Input: dimensioned drawing with shaded views. Units: mm. Origin: part minimum x, y, z. A direction names the side the tool comes from. Coordinates: 2 decimals unless noted, no trailing zeros. Order: outer loops, then holes, each group sorted by start corner. A loop starts at its lowest first (then second) coordinate and runs counter-clockwise, first axis right, second up.
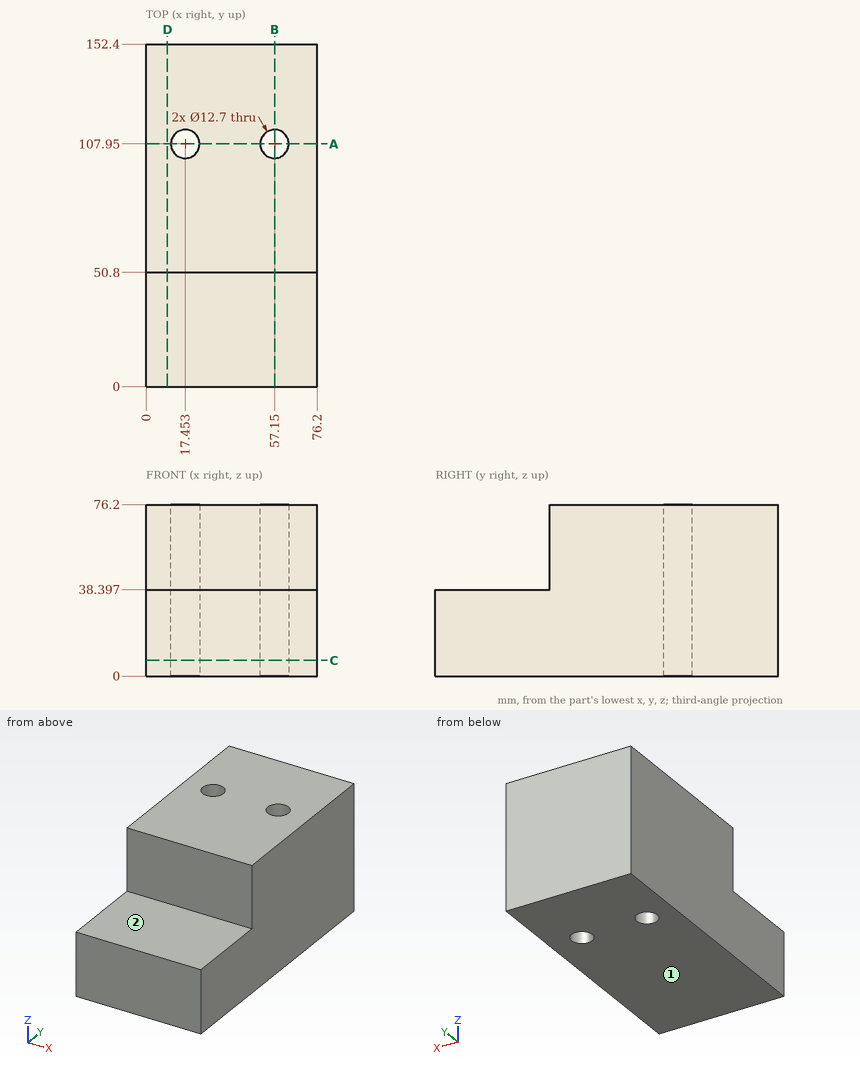
1. Material intervals for line 1 along X through (y, z) = (107, 26) (1 decimal); line 2 along Y through (x, z) = (57, 16); line 3 along Y through (x, z) = (39, 71.5), sorted ascending.
2. Section query D-D, the plane x = 9.5. Output: boundary loops of the cut face in (y, z), plus the area to 3 significant figures.
3. Access query for the marked faces 1 and 2. Directions: +Z, -Z, +X, -X, +Y, -Y. A direction counts if a zero-diameter tool reaches every point of the face in a straight line with its end or side. Return the directions, or none.
4. Section query A-A, the plane y = 107.95. Output: boundary loops of the cut face in (x, z).
5. Contact query for flat-ended pins moving along their axis: P1, Ø11.5, axis at x = 57.15, y = 107.95, coming from the -Z side; P2, Ø11.5, axis at x = 55, z = 51, coming from the -Y side; P3, Ø1.5, axis at x = 49, y = 48.5, coming from the +Z side. Output: stop coordinate, or through.
6. Section query C-C, the plane z = 7. Output: boundary loops of the cut face in (x, y), plus the area to 3 significant figures.
7. Section query B-B, the plane x = 57.15. Output: boundary loops of the cut face in (y, z).
Answer key:
1. line 1: x = 0 to 11.2, 23.7 to 50.9, 63.4 to 76.2
1. line 2: y = 0 to 101.6, 114.3 to 152.4
1. line 3: y = 50.8 to 152.4
2. outline: (0, 0) - (152.4, 0) - (152.4, 76.2) - (50.8, 76.2) - (50.8, 38.4) - (0, 38.4) - close
2. area: 9,690 mm2
3. face 1: -Z, +X, -X, +Y, -Y
3. face 2: +Z, +X, -X, -Y
4. outline: (0, 0) - (11.1, 0) - (11.1, 76.2) - (0, 76.2) - close; (23.8, 0) - (50.8, 0) - (50.8, 76.2) - (23.8, 76.2) - close; (63.5, 0) - (76.2, 0) - (76.2, 76.2) - (63.5, 76.2) - close
5. P1: passes through
5. P2: stops at y = 50.8
5. P3: stops at z = 38.4
6. outline: (0, 0) - (76.2, 0) - (76.2, 152.4) - (0, 152.4) - close; hole circle Ø12.7 at (17.45, 107.95); hole circle Ø12.7 at (57.15, 107.95)
6. area: 11,400 mm2
7. outline: (0, 0) - (101.6, 0) - (101.6, 76.2) - (50.8, 76.2) - (50.8, 38.4) - (0, 38.4) - close; (114.3, 0) - (152.4, 0) - (152.4, 76.2) - (114.3, 76.2) - close
